The listing builds one solid part. Answer for the finished solid, in the listing's coordinates (mm). Coordinates: 2 decimals unless noted, no trailing zeros. Order: outer loops, then holes, each group sorted by start corner. A loop starts at its lowest first (then second) coordinate and runs counter-clockwise, first axis right, second up. Notation, with made-up numbers: (59, 30) -> (112, 30) arc R25 cw to (112, 62) -> close; hole circle Ø2 at (86.5, 37). An arc over 180 degrees is marked (long way). Return JSON: item names as keys, results as strings.
```python
from build123d import *

# Parameters (mm, degrees)
SKETCH2_W          = 93
SKETCH2_H          = 198.84
EXTRUDE1_DEPTH     = 1.6
SKETCH3_W          = 2
SKETCH3_H          = 4.8
CUT_EXTRUDE1_DEPTH = 220.519715743
SKETCH4_W          = 35.6
SKETCH4_H          = 24
CUT_EXTRUDE2_DEPTH = 220.519715743
SKETCH6_W          = 25
SKETCH6_H          = 25
CUT_EXTRUDE3_DEPTH = 220.519715743
SKETCH7_R          = 1.25
CUT_EXTRUDE4_DEPTH = 220.519715743
SKETCH8_R          = 1.25
CUT_EXTRUDE5_DEPTH = 220.519715743
SKETCH10_W         = 1
SKETCH10_H         = 1.6
CUT_EXTRUDE6_DEPTH = 220.519715743


with BuildPart() as part:
    # Sketch2 → Extrude1 (new body)
    with BuildSketch(Plane(origin=(0, 0, 0), x_dir=(1, 0, 0), z_dir=(0, 1, 0))):
        with Locations((46.5, 99.42)):
            Rectangle(SKETCH2_W, SKETCH2_H)
    extrude(amount=EXTRUDE1_DEPTH)

    # Sketch3 → Cut-Extrude1 (cut, through all)
    with BuildSketch(Plane(origin=(0, 1.6, 0), x_dir=(-1, 0, 0), z_dir=(0, 1, 0))):
        with Locations((-1, -2.4)):
            Rectangle(SKETCH3_W, SKETCH3_H)
    extrude(amount=-CUT_EXTRUDE1_DEPTH, mode=Mode.SUBTRACT)

    # Sketch4 → Cut-Extrude2 (cut, through all)
    with BuildSketch(Plane(origin=(0, 1.6, 0), x_dir=(-1, 0, 0), z_dir=(0, 1, 0))):
        with Locations((-17.8, -100.6)):
            Rectangle(SKETCH4_W, SKETCH4_H)
    extrude(amount=-CUT_EXTRUDE2_DEPTH, mode=Mode.SUBTRACT)

    # Sketch6 → Cut-Extrude3 (cut, through all)
    with BuildSketch(Plane(origin=(0, 1.6, 0), x_dir=(-1, 0, 0), z_dir=(0, 1, 0))):
        with Locations((-12.5, -186.34)):
            Rectangle(SKETCH6_W, SKETCH6_H)
    extrude(amount=-CUT_EXTRUDE3_DEPTH, mode=Mode.SUBTRACT)

    # Sketch7 → Cut-Extrude4 (cut, through all)
    with BuildSketch(Plane(origin=(0, 1.6, 0), x_dir=(-1, 0, 0), z_dir=(0, 1, 0))):
        with Locations(Location((-29.077, -195.3, 0), (0, 0, 90))):
            Circle(SKETCH7_R)
        with Locations(Location((-86.077, -195.3, 0), (0, 0, 90))):
            Circle(SKETCH7_R)
        with Locations(Location((-4.2, -78.7, 0), (0, 0, 90))):
            Circle(SKETCH7_R)
        with Locations(Location((-86.077, -78.7, 0), (0, 0, 90))):
            Circle(SKETCH7_R)
    extrude(amount=-CUT_EXTRUDE4_DEPTH, mode=Mode.SUBTRACT)

    # Sketch8 → Cut-Extrude5 (cut, through all)
    with BuildSketch(Plane(origin=(0, 1.6, 0), x_dir=(-1, 0, 0), z_dir=(0, 1, 0))):
        with Locations(Location((-56, -21.4, 0), (0, 0, 90))):
            Circle(SKETCH8_R)
    extrude(amount=-CUT_EXTRUDE5_DEPTH, mode=Mode.SUBTRACT)

    # Sketch10 → Cut-Extrude6 (cut, through all)
    with BuildSketch(Plane(origin=(0, 0, -198.84), x_dir=(-1, 0, 0), z_dir=(0, 0, -1))):
        with Locations((-92.5, 0.8)):
            Rectangle(SKETCH10_W, SKETCH10_H)
    extrude(amount=-CUT_EXTRUDE6_DEPTH, mode=Mode.SUBTRACT)


solid = part.part
```
Item 1: The part is cut by section B-B on z = -92. Determine the outline of the cut face in (x, y).
Answer list:
{"outline": "(35.6, 0) -> (92, 0) -> (92, 1.6) -> (35.6, 1.6) -> close"}
Item 2: Flat-ended cylindrical pins translate along their axes: pin 1 (0.5 mm diameter, centred on x = 16, y = 1, fed in from -Z); pin 2 (0.5 mm diameter, centred on y = 1, z = -101, fed in from -X); pin 3 (0.5 mm diameter, centred on x = 0.5, y = 0.5, fed in from +Z); pin 4 (2 mm diameter, centred on x = 56, z = -21.4, fed in from -Y). Find the tip coordinate at first contact, or state that the pin passes through.
Answer list:
{"pin 1": "z = -173.84", "pin 2": "x = 35.6", "pin 3": "z = -4.8", "pin 4": "through"}
Item 3: The part is cut by section A-A on y = 1.2. Determine the outline of the cut face in (x, z), plus the area to 3 significant figures.
Answer list:
{"outline": "(0, -173.84) -> (25, -173.84) -> (25, -198.84) -> (92, -198.84) -> (92, 0) -> (2, 0) -> (2, -4.8) -> (0, -4.8) -> (0, -88.6) -> (35.6, -88.6) -> (35.6, -112.6) -> (0, -112.6) -> close; hole circle Ø2.5 at (4.2, -78.7); hole circle Ø2.5 at (29.08, -195.3); hole circle Ø2.5 at (56, -21.4); hole circle Ø2.5 at (86.08, -195.3); hole circle Ø2.5 at (86.08, -78.7)", "area": "16,800 mm2"}
Item 4: Find the intervals of material crossed by probe 1 along X at (y, z) = (1.15, -78.7); probe 2 along X at (y, z) = (0.5, -195.3); probe 3 along X at (y, z) = (0.7, -21.4), in increasing order.
Answer list:
{"probe 1": "0 to 2.95, 5.45 to 84.83, 87.33 to 92", "probe 2": "25 to 27.83, 30.33 to 84.83, 87.33 to 92", "probe 3": "0 to 54.75, 57.25 to 92"}
